The figure shows three views and two pictorial views of one solid part (mm, origin at its lowest corner). Answer the questions. A direction names the side the tool comes from. Give positions to 0.01 mm unless a question says otherwise; leave off trailing zeros. Order: outer loops, then holes, each group sorted by start corner. A loop starts at its lowest first (then second) coordinate and runs counter-clockwise, first axis right, second up. Notation, with made-up numbers: (-19, 62) - (28, 62) arc R21 ccw to (28, 80) - close; hole circle Ø6 at (-35.5, 32.25). An arc over 180 degrees is marked (long way). Write item = value, one per line.
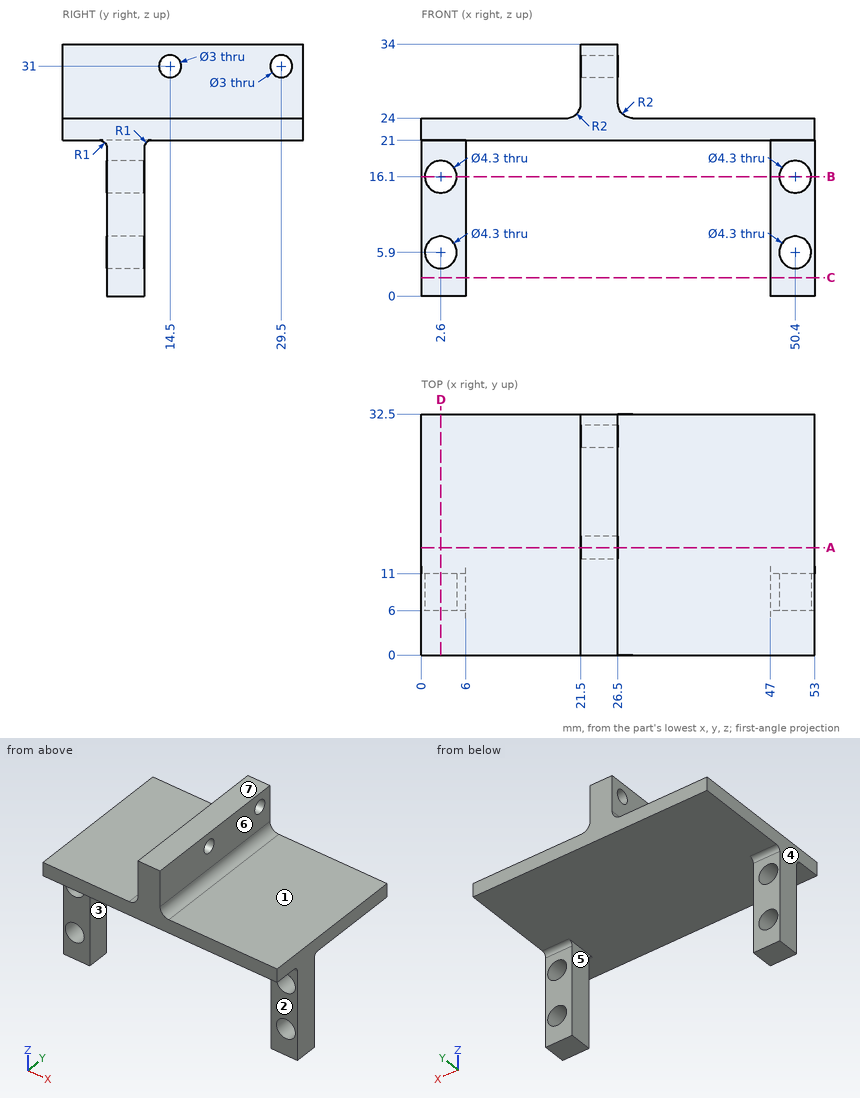
1. Section C-C (z = 2.5) is taken. Determine the outline of the cut face in (x, y), and give its area (3 significant figures).
Recorded:
outline = (0, 6) - (6, 6) - (6, 11) - (0, 11) - close; (47, 6) - (53, 6) - (53, 11) - (47, 11) - close
area = 60.0 mm^2
2. Section D-D (x = 2.6) is taken. Determine the outline of the cut face in (y, z).
Recorded:
outline = (0, 21) - (5, 21) arc R1 cw to (6, 20) - (6, 18.25) - (11, 18.25) - (11, 20) arc R1 cw to (12, 21) - (32.5, 21) - (32.5, 24) - (0, 24) - close; (6, 0) - (11, 0) - (11, 3.75) - (6, 3.75) - close; (6, 8.05) - (11, 8.05) - (11, 13.95) - (6, 13.95) - close
3. Section B-B (z = 16.1) is taken. Determine the outline of the cut face in (x, y).
Recorded:
outline = (0, 6) - (0.45, 6) - (0.45, 11) - (0, 11) - close; (4.75, 6) - (6, 6) - (6, 11) - (4.75, 11) - close; (47, 6) - (48.25, 6) - (48.25, 11) - (47, 11) - close; (52.55, 6) - (53, 6) - (53, 11) - (52.55, 11) - close
4. Straight lines are drawn through the part: L1, parallel to X at y = 9, z = 16; L2, parallel to Z at x = 2, y = 7; L3, parallel to Z at x = 23.9, y = 14.5. For each, find the intervals that lie inside material, in ascending order. Write a range as [from, to].
Recorded:
L1 = [0, 0.45], [4.75, 6], [47, 48.25], [52.55, 53]
L2 = [0, 3.84], [7.96, 14.04], [18.16, 24]
L3 = [21, 29.5], [32.5, 34]
5. Flat-ended cylindrical pins translate along their axes: pin 1 (6.5 mm diameter, centred on x = 49, z = 6, fed in from -Y); pin 2 (4 mm diameter, centred on x = 9, y = 7.5, fed in from -Z); pin 3 (5.5 mm diameter, centred on x = 2.6, z = 5.9, fed in from +Y); pin 4 (4 mm diameter, centred on x = 2.6, z = 16.1, fed in from +Y). Find the tip coordinate at first contact, or state that the pin passes through.
Recorded:
pin_1 = 6
pin_2 = 21
pin_3 = 11
pin_4 = through
6. For the marked faces 1, 2 and 3, determine the directions among +Z, -Z, +X, -X, +Y, -Y from which every point of the face is accessible in a straight line to the end or side of a thin tool.
Recorded:
face_1 = +Z, +X, +Y, -Y
face_2 = -Z, +X, -X, -Y
face_3 = -Z, +Y, -Y
7. Determine the mould class of the marked faces 4, 5, 6 and 7 for opening direction X: +X half, -X half, draft (parallel to the pull), parting line (faces both ways), or undercut.
Recorded:
face_4 = -X half
face_5 = undercut
face_6 = +X half
face_7 = draft
8. Section A-A (y = 14.5) is taken. Determine the outline of the cut face in (x, z).
Recorded:
outline = (0, 21) - (53, 21) - (53, 24) - (28.5, 24) arc R2 cw to (26.5, 26) - (26.5, 29.5) - (21.5, 29.5) - (21.5, 26) arc R2 cw to (19.5, 24) - (0, 24) - close; (21.5, 32.5) - (26.5, 32.5) - (26.5, 34) - (21.5, 34) - close
